```python
from build123d import *

# Parameters (mm, degrees)
F1_DEPTH = 63.5
F0_W     = 25.3651374038
F0_H     = 19.05
F2_DEPTH = 25.4
F3_DEPTH = 7.9375
F0_W_2   = 25.4
F0_H_2   = 28.575
F5_R     = 6.35


with BuildPart() as f1:
    # F0 (on Front) → F1 (new body, symmetric)
    with BuildSketch(Plane.XZ):
        Polygon((36.9096121311, 9.525), (-55.9596121311, 9.525), (-55.9596121311, -9.525), (55.9596121311, -9.525), (55.9596121311, 9.525), align=None)
    extrude(amount=F1_DEPTH, both=True)

    # F0 (on Front) → F2 (join, symmetric)
    with BuildSketch(Plane.XZ):
        with BuildLine():
            Line((36.9096121311, 27.0002), (36.9096121311, 9.525))
            Line((36.9096121311, 9.525), (55.9596121311, 9.525))
            Line((55.9596121311, 9.525), (55.9596121311, 27.0002))
            ThreePointArc((55.9596121311, 27.0002), (60.6092919798, 38.2255201513), (71.8346121311, 42.8752))
            Line((71.8346121311, 42.8752), (100.552007556, 42.8752))
            Line((100.552007556, 42.8752), (100.552007556, 61.9252))
            Line((100.552007556, 61.9252), (71.8346121311, 61.9252))
            ThreePointArc((71.8346121311, 61.9252), (47.1389077982, 51.6959043329), (36.9096121311, 27.0002))
        make_face()
        with Locations((113.2345762579, 52.4002)):
            Rectangle(F0_W, F0_H)
    extrude(amount=F2_DEPTH, both=True)

    # F0 (on Front) → F3 (join, symmetric)
    with BuildSketch(Plane.XZ):
        with BuildLine():
            add(Edge.make_bspline(
                [(-55.9596121311, 9.525), (-43.233461678, 61.7118962109), (17.0044116676, 79.1671946645), (71.8346121311, 61.9252)],
                knots=[0, 0, 0, 0, 138.1200373401, 138.1200373401, 138.1200373401, 138.1200373401], degree=3))
            Line((-55.9596121311, 9.525), (36.9096121311, 9.525))
            Line((36.9096121311, 9.525), (36.9096121311, 27.0002))
            ThreePointArc((36.9096121311, 27.0002), (47.1389077982, 51.6959043329), (71.8346121311, 61.9252))
        make_face()
    extrude(amount=F3_DEPTH, both=True)

    # F0 (on Front) → F4 (revolve)
    with BuildSketch(Plane.XZ):
        with Locations((138.652007556, 52.3875)):
            Rectangle(F0_W_2, F0_H_2)
    revolve(axis=Axis((125.952007556, 0, 52.3875), (0, 0, -1)))

    # F5
    f5_edges = [f1.edges().sort_by_distance(p)[0] for p in [
        (-55.959612, -63.5, 0),
        (55.959612, -63.5, 0),
        (55.959612, 63.5, 0),
        (-55.959612, 63.5, 0),
    ]]
    fillet(f5_edges, radius=F5_R)


solid = f1.part
```
Verification items for the finished model (mm, model axes). A direction names the side the tool comes from. Give positions to 0.01 mm unless a question says otherwise; leave off trailing zeros. Loops run counter-clockwise (first coordinate to the right, second up) from the corner with the lowest first, then second, coordinate; pieces in that order, holes last.
1. Section check C-C, the plane x = 76. Enter the section's corners in (y, z).
2. Section check A-A, the plane z = 7. Enter the section's corners in (x, y).
3. Thickness scan on line 1 (X direction, y = -55.5, z = 6); line 2 (Z direction, x = 26, y = 33) (3 decimals); line 3 (Y direction, x = 13.5, z = 26.5). Record the ranges inside material, lowest first.
4. Set-up check for faces 1 (the flat face through (126, 0, 66.675)), 2 (the flat face through (55.96, -1, 4)), 3 (the flat face through (71, 25.4, 48)), 4 (the flat face through (-5, 7.938, 37)), 5 (the cylindrical face through (60.487, -0.356, 38.101)): record each of +Z, -Z, +X, -X, +Y, -Y from which the full face is reachable in a straight line by a thin tool's end or side.
5. Section check D-D, the plane y = 41.5. Enter the section's corners in (x, z) (3 decimals).
6. Go/stop test with flat-tipped pins: pin 1 Ø15 at (x, y) = (120, 1) entering from +Z (3 decimals); pin 2 Ø3 at (y, z) = (0, 40.5) entering from -X; pin 3 Ø2 at (y, z) = (-4.5, 40.5) entering from -X; pin 4 Ø19 at (y, z) = (20.5, 17) entering from -X. Record where each tip stops, or that it passes through.
7. Section check B-B, the plane y = 13.5. Enter the section's corners in (x, z) (3 decimals), then the cut area to 3 significant figures.
Geometry says:
1. outline: (-25.4, 42.88) - (25.4, 42.88) - (25.4, 61.93) - (-25.4, 61.93) - close
2. outline: (-55.96, -57.15) arc R6.35 ccw to (-49.61, -63.5) - (49.61, -63.5) arc R6.35 ccw to (55.96, -57.15) - (55.96, 57.15) arc R6.35 ccw to (49.61, 63.5) - (-49.61, 63.5) arc R6.35 ccw to (-55.96, 57.15) - close
3. line 1: x = -55.96 to 55.96
3. line 2: z = -9.525 to 9.525
3. line 3: y = -7.94 to 7.94
4. face 1: +Z, +X, +Y, -Y
4. face 2: -Z, +X, +Y, -Y
4. face 3: +Z, +X, -X, +Y
4. face 4: +Z, -X, +Y
4. face 5: -Z, +Y, -Y
5. outline: (-55.96, -9.525) - (55.96, -9.525) - (55.96, 9.525) - (-55.96, 9.525) - close
6. pin 1: stops at z = 66.675
6. pin 2: stops at x = -41.16
6. pin 3: stops at x = -40.74
6. pin 4: stops at x = -55.96
7. outline: (-55.96, -9.525) - (55.96, -9.525) - (55.96, 27) arc R15.875 cw to (71.835, 42.875) - (104.437, 42.875) - (104.437, 38.1) - (147.467, 38.1) - (147.467, 66.675) - (104.437, 66.675) - (104.437, 61.925) - (71.835, 61.925) arc R34.925 ccw to (36.91, 27) - (36.91, 9.525) - (-55.96, 9.525) - close
7. area: 5,080 mm2
